```python
from build123d import *

# Parameters (mm, degrees)
SKETCH2_W          = 44.887778639
SKETCH2_H          = 40.820436252
CUT_EXTRUDE1_DEPTH = 151.069983674
CUT_EXTRUDE2_DEPTH = 151.069983674
SKETCH5_R          = 3.75
CUT_EXTRUDE3_DEPTH = 133.664991614
CUT_EXTRUDE4_DEPTH = 151.069983674
CUT_EXTRUDE5_DEPTH = 10
FILLET1_R          = 1


with BuildPart() as part:
    # Sketch1 → Revolve1 (revolve)
    with BuildSketch(Plane.XY, mode=Mode.PRIVATE) as revolve1_sk:
        with BuildLine():
            Line((0, 0), (139, 0))
            Line((139, 0), (139, 25))
            Line((139, 25), (122, 25))
            ThreePointArc((122, 25), (120.585786438, 25.585786438), (120, 27))
            Line((120, 27), (120, 40))
            Line((120, 40), (91.5, 40))
            Line((91.5, 40), (89, 37.5))
            Line((89, 37.5), (50, 37.5))
            Line((50, 37.5), (47.5, 40))
            Line((47.5, 40), (19, 40))
            Line((19, 40), (19, 27))
            ThreePointArc((19, 27), (18.414213562, 25.585786438), (17, 25))
            Line((17, 25), (0, 25))
            Line((0, 25), (0, 0))
        make_face()
    revolve(revolve1_sk.sketch.rotate(Axis((0, 0, 0), (1, 0, 0)), 90), axis=Axis((0, 0, 0), (1, 0, 0)))

    # Sketch2 → Cut-Extrude1 (cut, through all)
    with BuildSketch(Plane.ZY):
        with Locations((22.44388932, 20.410218126)):
            Rectangle(SKETCH2_W, SKETCH2_H)
    extrude(amount=-CUT_EXTRUDE1_DEPTH, mode=Mode.SUBTRACT)

    # Sketch4 → Cut-Extrude2 (cut, through all)
    with BuildSketch(Plane.ZY):
        with BuildLine():
            Line((0, 4), (-12, 4))
            ThreePointArc((-12, 4), (-15, 7), (-12, 10))
            Line((-12, 10), (0, 10))
            ThreePointArc((0, 10), (3, 7), (0, 4))
        make_face()
    extrude(amount=-CUT_EXTRUDE2_DEPTH, mode=Mode.SUBTRACT)

    # Sketch5 → Cut-Extrude3 (cut, through all)
    with BuildSketch(Plane.ZY.offset(-19)):
        with Locations((-8.282209443, 30.909626441)):
            Circle(SKETCH5_R)
        with Locations((-22.62297233, 22.626635765)):
            Circle(SKETCH5_R)
        with Locations((-30.901659317, 8.283387998)):
            Circle(SKETCH5_R)
        with Locations((-30.90041693, -8.277572517)):
            Circle(SKETCH5_R)
        with Locations((-22.619578006, -22.619578006)):
            Circle(SKETCH5_R)
        with Locations((-8.277572517, -30.90041693)):
            Circle(SKETCH5_R)
        with Locations((8.283387998, -30.901659317)):
            Circle(SKETCH5_R)
        with Locations((22.626635765, -22.62297233)):
            Circle(SKETCH5_R)
        with Locations((30.909626441, -8.282209443)):
            Circle(SKETCH5_R)
    extrude(amount=-CUT_EXTRUDE3_DEPTH, mode=Mode.SUBTRACT)

    # Sketch6 → Cut-Extrude4 (cut, through all)
    with BuildSketch(Plane(origin=(0, 0, 0), x_dir=(1, 0, 0), z_dir=(0, 1, 0))):
        with BuildLine():
            Line((107.279227454, -25.208360839), (111.810766389, -27.321452148))
            ThreePointArc((111.810766389, -27.321452148), (157.26284287, -63.800600209), (133.79055467, -10.45576741))
            Line((133.79055467, -10.45576741), (132.922313782, -5.531728645))
            ThreePointArc((132.922313782, -5.531728645), (117.693349985, -12.23263309), (107.279227454, -25.208360839))
        make_face()
    extrude(amount=-CUT_EXTRUDE4_DEPTH, mode=Mode.SUBTRACT)

    # Sketch7 → Cut-Extrude5 (cut)
    with BuildSketch(Plane.ZY):
        with BuildLine():
            Line((-4, 0), (-21, 0))
            ThreePointArc((-21, 0), (-2.009217424, -20.903661051), (20.615528128, -4))
            Line((20.615528128, -4), (-4, -4))
            Line((-4, -4), (-4, 0))
        make_face()
    extrude(amount=-CUT_EXTRUDE5_DEPTH, mode=Mode.SUBTRACT)

    # Fillet1
    fillet1_edges = [part.edges().sort_by_distance(p)[0] for p in [
        (10, -2, -4),
        (10, -4, 8.307764064),
        (10, -20.903661051, -2.009217424),
        (10, 0, -12.5),
        (0, -2, -4),
        (0, 0, -12.5),
        (0, -20.903661051, -2.009217424),
        (0, -4, 8.307764064),
    ]]
    fillet(fillet1_edges, radius=FILLET1_R)


solid = part.part
```
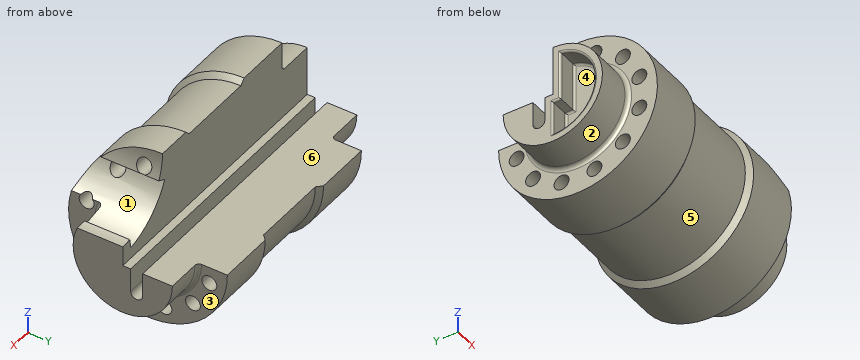
Geometry check sheet. Reference: the model listing, model coordinates, mm. Face numbers are marked on the shaded views. A direction names the side the tool comes from. Give positions to 0.01 mm unless a question says otherwise; leave off trailing zeros.
1) Access from +Z, -Z, +X, -X, +Y, -Y to the whole of each face (thin tool, end or side, straight path). Record for the marked faces 4, 5 and 6.
2) Release check for a two-part mould opening along Z. For the marked faces 1, 2 and 3 record: pulls with the +Z half, pulls with the -Z half, needs draft (parallel to the pull), parting line crosses it, or undercut.
3) Gauge pin test, flat ends, axial feed: pin 1 (12 mm diameter, centred on x = 112.5, z = -27.5, fed in from -Y); pin 2 (4 mm diameter, centred on x = 56, z = 28, fed in from -Y); pin 3 (9.5 mm diameter, centred on x = 40, z = -8, fed in from -Y). Record the tip position at first contact, or that the pin passes through.
4) Material ranges on L1, parallel to Y at x = 44, z = -28.5; L2, parallel to Z at x = 54.5, y = -22; L3, parallel to Y at x = 75.5, z = -8, recorded low to high.
5) Section check A-A, the plane x = 38.5. State how many separate pieces and enclosed holes the cut face has, and give its area (3 significant figures).
Computed:
1. face 4: -X
1. face 5: none
1. face 6: +Z, +X, -X, +Y
2. face 1: undercut
2. face 2: parting line crosses it
2. face 3: needs draft
3. pin 1: stops at y = -33.73
3. pin 2: stops at y = -27.02
3. pin 3: stops at y = -39.87
4. L1: y = -28.07 to -11.16, -5.4 to 5.4, 11.16 to 28.07
4. L2: z = -30.37 to -26.32, -18.92 to 18.93, 26.32 to 30.37
4. L3: y = -36.64 to -34.64, -27.16 to 4, 10 to 27.17, 34.65 to 36.64
5. separate pieces: 1
5. enclosed holes: 9
5. area: 3,290 mm2
